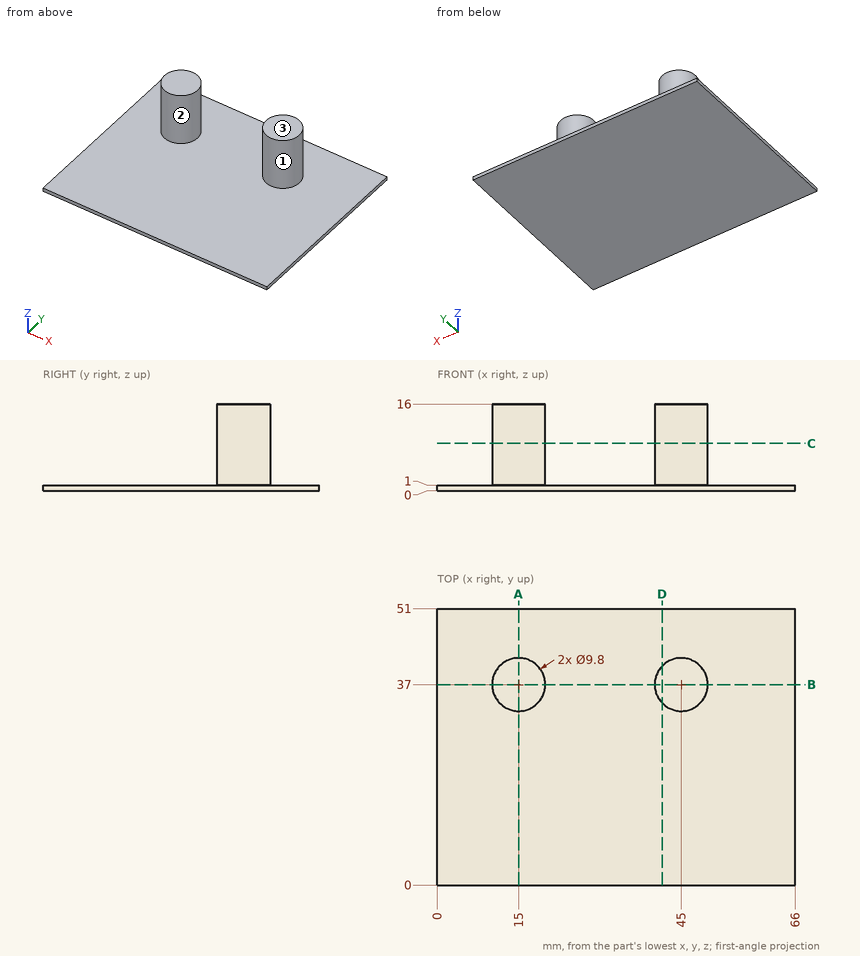
Verification items for this drawing (mm, ordinates from the low corner). Coordinates: 2 decimals unless noted, no trailing zeros. Loops run counter-clockwise (first coordinate to the right, second up) from the corner with the lowest first, then second, coordinate; pieces in that order, holes last. Notation, with made-up numbers: (-22, 85.5) - (-3, 85.5) arc R32 ccw to (-3, 122.5) - close; hole circle Ø10 at (-20.75, 21.25). An arc over 180 degrees is marked (long way). Answer as a JSON object with one key per item and string values.
(1) Cross-section at B-B, the plane y = 37. Record the boundary of the cut face in (x, z), then the cut area to 3 significant figures.
Response:
{"outline": "(0, 0) - (66, 0) - (66, 1) - (49.9, 1) - (49.9, 16) - (40.1, 16) - (40.1, 1) - (19.9, 1) - (19.9, 16) - (10.1, 16) - (10.1, 1) - (0, 1) - close", "area": "360 mm²"}
(2) Cross-section at C-C, the plane z = 8.75. Record the boundary of the cut face in (x, y).
Response:
{"outline": "circle Ø9.8 at (15, 37); circle Ø9.8 at (45, 37)"}
(3) Go/stop test with flat-tipped pins: pin 1 Ø3 at (x, z) = (43, 4.5) entering from -Y; pin 2 Ø2 at (x, z) = (43.5, 12.5) entering from +Y; pin 3 Ø4 at (x, y) = (56.5, 8.5) entering from +Z. Record where each tip stops, or that it passes through.
Response:
{"pin 1": "stops at y = 32.13", "pin 2": "stops at y = 41.87", "pin 3": "stops at z = 1"}
(4) Mould release check, pull along X, two halves, no side actions. Record for the marked faces 1, 2 and 3: pulls with the +X half, pulls with the -X half, needs draft (parallel to the pull), parting line crosses it, or undercut.
Response:
{"face 1": "undercut", "face 2": "undercut", "face 3": "needs draft"}
(5) Scan lines: line 1 along Z through (x, y) = (26, 16.5); line 2 along X through (y, z) = (33, 7.5); line 3 along X through (y, z) = (39, 4.5). Record each from-to range of solid material in increasing order.
Response:
{"line 1": "z = 0 to 1", "line 2": "x = 12.17 to 17.83, 42.17 to 47.83", "line 3": "x = 10.53 to 19.47, 40.53 to 49.47"}
(6) Cross-section at D-D, the plane x = 41.5. Record the boundary of the cut face in (y, z), then the cut area to 3 significant figures.
Response:
{"outline": "(0, 0) - (51, 0) - (51, 1) - (40.43, 1) - (40.43, 16) - (33.57, 16) - (33.57, 1) - (0, 1) - close", "area": "154 mm²"}
(7) Cross-section at A-A, the plane x = 15. Record the boundary of the cut face in (y, z).
Response:
{"outline": "(0, 0) - (51, 0) - (51, 1) - (41.9, 1) - (41.9, 16) - (32.1, 16) - (32.1, 1) - (0, 1) - close"}
